```python
from build123d import *

# Parameters (mm, degrees)
SKETCH1_W                       = 20.45
SKETCH1_H                       = 18.1
BOSS_EXTRUDE2_DEPTH             = 1
BOSS_EXTRUDE3_REACH             = 15.691
BOSS_EXTRUDE3_DIRECTION_2_REACH = 15.691
SKETCH4_R                       = 1.65
CUT_EXTRUDE1_DEPTH              = 5
SKETCH6_R                       = 2.75
CUT_EXTRUDE2_DEPTH              = 4
SKETCH7_R                       = 1.15
CUT_EXTRUDE3_DEPTH              = 9.05
SKETCH8_R                       = 2
CUT_EXTRUDE4_DEPTH              = 8
CUT_EXTRUDE4_DIRECTION_2_REACH  = 16.541
FILLET2_R                       = 1
FILLET3_R                       = 0.8


with BuildPart() as part:
    # Sketch1 → Boss-Extrude2 (new body)
    with BuildSketch(Plane(origin=(0, 0, 0), x_dir=(1, 0, 0), z_dir=(0, 1, 0))):
        Rectangle(SKETCH1_W, SKETCH1_H)
    extrude(amount=BOSS_EXTRUDE2_DEPTH)

    # Boss-Extrude3: up to this face of the body (flat: up to its plane)
    boss_extrude3_end = Plane(part.part.faces().sort_by_distance((10.225, 0.5, 0))[0])
    # Sketch3 → Boss-Extrude3 (add, up to the picked face)
    with BuildSketch(Plane(origin=(0, 0, 0), x_dir=(0, 0, -1), z_dir=(1, 0, 0)), mode=Mode.PRIVATE) as boss_extrude3_sk1:
        Polygon((9.05, 1), (9.05, 5), (7.05, 5), (3.05, 1), align=None)
    boss_extrude3_tool1 = split(extrude(boss_extrude3_sk1.sketch, amount=BOSS_EXTRUDE3_REACH, mode=Mode.PRIVATE), bisect_by=boss_extrude3_end, keep=Keep.BOTH, mode=Mode.PRIVATE)
    add(boss_extrude3_tool1.solids().sort_by(Axis((0, 2.666667, -6.883333), (1, 0, 0)))[0])

    # Boss-Extrude3 direction 2: up to this face of the body (flat: up to its plane)
    boss_extrude3_direction_2_end = Plane(part.part.faces().sort_by_distance((-10.225, 0.5, 0))[0])
    # Sketch3 → Boss-Extrude3 direction 2 (add, up to the picked face)
    with BuildSketch(Plane(origin=(0, 0, 0), x_dir=(0, 0, -1), z_dir=(1, 0, 0)), mode=Mode.PRIVATE) as boss_extrude3_direction_2_sk1:
        Polygon((9.05, 1), (9.05, 5), (7.05, 5), (3.05, 1), align=None)
    boss_extrude3_direction_2_tool1 = split(extrude(boss_extrude3_direction_2_sk1.sketch, amount=-BOSS_EXTRUDE3_DIRECTION_2_REACH, mode=Mode.PRIVATE), bisect_by=boss_extrude3_direction_2_end, keep=Keep.BOTH, mode=Mode.PRIVATE)
    add(boss_extrude3_direction_2_tool1.solids().sort_by(Axis((0, 2.666667, -6.883333), (-1, 0, 0)))[0])

    # Sketch4 → Cut-Extrude1 (cut)
    with BuildSketch(Plane(origin=(0, 5, 0), x_dir=(1, 0, 0), z_dir=(0, 1, 0))):
        with Locations(Location((-5.505, 5.45, 0), (0, 0, 104.141110234))):
            Circle(SKETCH4_R)
        with Locations(Location((5.505, 5.45, 0), (0, 0, 75.858889766))):
            Circle(SKETCH4_R)
    extrude(amount=-CUT_EXTRUDE1_DEPTH, mode=Mode.SUBTRACT)

    # Sketch6 → Cut-Extrude2 (cut)
    with BuildSketch(Plane(origin=(0, 5, 0), x_dir=(1, 0, 0), z_dir=(0, 1, 0))):
        with Locations((-5.505, 5.45)):
            Circle(SKETCH6_R)
        with Locations((5.505, 5.45)):
            Circle(SKETCH6_R)
    extrude(amount=-CUT_EXTRUDE2_DEPTH, mode=Mode.SUBTRACT)

    # Sketch7 → Cut-Extrude3 (cut)
    with BuildSketch(Plane.XY):
        with Locations((0, 2.5)):
            Circle(SKETCH7_R)
    extrude(amount=-CUT_EXTRUDE3_DEPTH, mode=Mode.SUBTRACT)

    # Sketch8 → Cut-Extrude4 (cut)
    with BuildSketch(Plane.XY):
        with Locations(Location((0, 2.5, 0), (0, 0, 228.590377891))):
            Circle(SKETCH8_R)
    extrude(amount=-CUT_EXTRUDE4_DEPTH, mode=Mode.SUBTRACT)

    # Cut-Extrude4 direction 2: up to this face of the body (flat: up to its plane)
    cut_extrude4_direction_2_end = Plane(part.part.faces().sort_by_distance((0, 0.5, 9.05))[0])
    # Sketch8 → Cut-Extrude4 direction 2 (cut, up to the picked face)
    with BuildSketch(Plane.XY, mode=Mode.PRIVATE) as cut_extrude4_direction_2_sk1:
        with Locations(Location((0, 2.5, 0), (0, 0, 228.590377891))):
            Circle(SKETCH8_R)
    cut_extrude4_direction_2_tool1 = split(extrude(cut_extrude4_direction_2_sk1.sketch, amount=CUT_EXTRUDE4_DIRECTION_2_REACH, mode=Mode.PRIVATE), bisect_by=cut_extrude4_direction_2_end, keep=Keep.BOTH, mode=Mode.PRIVATE)
    add(cut_extrude4_direction_2_tool1.solids().sort_by(Axis((0, 2.5, 0), (0, 0, 1)))[0], mode=Mode.SUBTRACT)

    # Fillet2
    fillet2_edges = [part.edges().sort_by_distance(p)[0] for p in [
        (10.225, 0.5, 9.05),
        (-10.225, 0.5, 9.05),
    ]]
    fillet(fillet2_edges, radius=FILLET2_R)

    # Fillet3
    # the kernel refuses this fillet: 0.8 mm, written as the material it adds along each edge
    with BuildSketch(Plane(origin=(-6.019145033, 1, -3.05), x_dir=(0, 0, 1), z_dir=(-1, 0, 0))) as fillet3_piece_1_section:
        with BuildLine():
            CenterArc((FILLET3_R * 0.414213562373, FILLET3_R), FILLET3_R, 225, 45)
            Line((-FILLET3_R * 0.292893218813, FILLET3_R * 0.292893218813), (0, 0))
            Line((0, 0), (FILLET3_R * 0.414213562373, 0))
        make_face()
    fillet3_piece_1 = extrude(amount=4.205854967, mode=Mode.PRIVATE)
    fillet3_piece_1 = fillet3_piece_1 - Plane(origin=(-5.505, 1.04586757, -5.45), x_dir=(1, 0, 0), z_dir=(0, 1, 0)) * Cylinder(2.75, 10, mode=Mode.PRIVATE)
    add(fillet3_piece_1)
    with BuildSketch(Plane(origin=(-0.494448531, 1, -3.05), x_dir=(0, 0, 1), z_dir=(-1, 0, 0))) as fillet3_piece_2_section:
        with BuildLine():
            CenterArc((FILLET3_R * 0.414213562373, FILLET3_R), FILLET3_R, 225, 45)
            Line((-FILLET3_R * 0.292893218813, FILLET3_R * 0.292893218813), (0, 0))
            Line((0, 0), (FILLET3_R * 0.414213562373, 0))
        make_face()
    fillet3_piece_2 = extrude(amount=4.496406436, mode=Mode.PRIVATE)
    fillet3_piece_2 = fillet3_piece_2 - Plane(origin=(-5.505, 1.043873753, -5.45), x_dir=(1, 0, 0), z_dir=(0, 1, 0)) * Cylinder(2.75, 11, mode=Mode.PRIVATE)
    fillet3_piece_2 = fillet3_piece_2 - Plane(origin=(0, 2.5, -3.015215502), x_dir=(-0.6614378277626023, -0.7500000000031267, 0), z_dir=(0, 0, 1)) * Cylinder(2, 11, mode=Mode.PRIVATE)
    add(fillet3_piece_2)
    with BuildSketch(Plane(origin=(4.990854967, 1, -3.05), x_dir=(0, 0.7071067811865468, -0.7071067811865482), z_dir=(-1, 0, 0))) as fillet3_piece_3_section:
        with BuildLine():
            CenterArc((FILLET3_R * 0.414213562373, -FILLET3_R), FILLET3_R, 90, 45)
            Line((-FILLET3_R * 0.292893218813, -FILLET3_R * 0.292893218813), (0, 0))
            Line((0, 0), (FILLET3_R * 0.414213562373, 0))
        make_face()
    fillet3_piece_3 = extrude(amount=4.496406436, mode=Mode.PRIVATE)
    fillet3_piece_3 = fillet3_piece_3 - Plane(origin=(0, 2.5, -3.015215403), x_dir=(-0.6614378277626023, -0.7500000000031267, 0), z_dir=(0, 0, 1)) * Cylinder(2, 11, mode=Mode.PRIVATE)
    fillet3_piece_3 = fillet3_piece_3 - Plane(origin=(5.505, 1.043873896, -5.45), x_dir=(1, 0, 0), z_dir=(0, 1, 0)) * Cylinder(2.75, 11, mode=Mode.PRIVATE)
    add(fillet3_piece_3)
    with BuildSketch(Plane(origin=(10.225, 1, -3.05), x_dir=(0, 0, 1), z_dir=(-1, 0, 0))) as fillet3_piece_4_section:
        with BuildLine():
            CenterArc((FILLET3_R * 0.414213562373, FILLET3_R), FILLET3_R, 225, 45)
            Line((-FILLET3_R * 0.292893218813, FILLET3_R * 0.292893218813), (0, 0))
            Line((0, 0), (FILLET3_R * 0.414213562373, 0))
        make_face()
    fillet3_piece_4 = extrude(amount=4.205854967, mode=Mode.PRIVATE)
    fillet3_piece_4 = fillet3_piece_4 - Plane(origin=(5.505, 1.045867594, -5.45), x_dir=(1, 0, 0), z_dir=(0, 1, 0)) * Cylinder(2.75, 10, mode=Mode.PRIVATE)
    add(fillet3_piece_4)


solid = part.part
```
Geometry check sheet. Reference: the model listing, model coordinates, mm. A direction names the side the tool comes from. Give positions to 0.01 mm unless a question says otherwise; leave off trailing zeros. Loops run counter-clockwise (first coordinate to the right, second up) from the corner with the lowest first, then second, coordinate; pieces in that order, holes last. Notation, with made-up numbers: M 12.5,32 L 36.5,32 A29 cw 36.5,67 Z; hole C 57.5,-38 d1. An arc over 180 degrees is marked long. Write item = value, one per line.
(1) Sectioned sample at A-A, the plane y = 2.5. Record the cut outline in (x, z) (3 decimals), plus the area to 3 significant figures.
Answer below:
outline = M -10.225,-9.05 L -1.15,-9.05 L -1.15,-8 L -2,-8 L -2,-4.55 L -2.906,-4.55 A2.75 cw long -8.104,-4.55 L -10.225,-4.55 Z; M 1.15,-9.05 L 10.225,-9.05 L 10.225,-4.55 L 8.104,-4.55 A2.75 cw long 2.906,-4.55 L 2,-4.55 L 2,-8 L 1.15,-8 Z
area = 42.3 mm2
(2) Sectioned sample at B-B, the plane x = 0. Record the cut outline in (y, z).
Answer below:
outline = M 0,-9.05 L 1.35,-9.05 L 1.35,-8 L 0.5,-8 L 0.5,9.05 L 0,9.05 Z; M 3.65,-9.05 L 5,-9.05 L 5,-7.05 L 4.5,-6.55 L 4.5,-8 L 3.65,-8 Z
(3) Tool access check on faces 1 (the face through (-0.84, 1.5, -8)), 2 (the face through (6, 1, 2)), 3 (the face through (-9.03, 3.14, -5.19)). Record the directions out of +Z, -Z, +X, -X, +Y, -Y that give a thin tool (end or side, any length) a straight path to the whole face; none if there is none.
Answer below:
face_1 = +Z
face_2 = +Y
face_3 = +Z, +X, -X, +Y
(4) Release check for a two-part mould opening along Y. For faces 4 (the face through (-0.249, 1.377, -8.518)), 5 (the face through (-10.225, 1, -4)), 6 (the face through (0, 5, -8)) record: released by +Y, released by -Y, zero draft, split by the parting line, or undercut.
Answer below:
face_4 = undercut
face_5 = zero draft
face_6 = released by +Y
(5) Sectioned sample at C-C, the plane z = -5.45. Record the cut outline in (x, y) (3 decimals).
Answer below:
outline = M -10.225,0 L -7.155,0 L -7.155,1 L -8.255,1 L -8.255,3.4 L -10.225,3.4 Z; M -3.855,0 L 3.855,0 L 3.855,1 L 2.755,1 L 2.755,3.4 L 1.786,3.4 A2 cw long -1.786,3.4 L -2.755,3.4 L -2.755,1 L -3.855,1 Z; M 7.155,0 L 10.225,0 L 10.225,3.4 L 8.255,3.4 L 8.255,1 L 7.155,1 Z
(6) Sectioned sample at D-D, the plane z = -0.25. Record the cut outline in (x, y) (3 decimals).
Answer below:
outline = M -10.225,0 L 10.225,0 L 10.225,1 L 1.323,1 A2 cw -1.323,1 L -10.225,1 Z
(7) Gauge pin test, flat ends, axial feed: pin 1 Ø1 at (x, z) = (1.5, 5) entering from -Y; pin 2 Ø10 at (x, z) = (6.5, 2.5) entering from +Y; pin 3 Ø2.5 at (x, z) = (-6, -2.5) entering from +Y; pin 4 Ø1.2 at (x, y) = (0.5, 2) entering from +Z. Record the tip position at first contact, or that the pin passes through.
Answer below:
pin_1 = 0
pin_2 = 1
pin_3 = 1.14
pin_4 = -8
(8) Material ranges on line 1 (Y direction, x = -7.5, z = 1.5); line 2 (X direction, y = 2, z = -5.45) (1 decimal); line 3 (X direction, y = 2.95, z = -7) (3 decimals), recorded low to high. Write a range as [from, to].
Answer below:
line_1 = [0, 1]
line_2 = [-10.2, -8.3], [-2.8, -1.9], [1.9, 2.8], [8.3, 10.2]
line_3 = [-10.225, -7.777], [-3.233, -1.949], [1.949, 3.233], [7.777, 10.225]
